For this review, use the dimensioned drawing (mm, ordinates from the lowest corner) and the shaded views. Give positions to 0.01 mm unless a question says otherwise; leave off trailing zeros. Loops run counter-clockwise (first coordinate to the right, second up) from the corner with the lowest first, then second, coordinate; pieces in that order, holes last. Notation, with made-up numbers: (-10, -8.5) -> (-1, -8.5) arc R33 ccw to (-1, 29.5) -> close; hole circle Ø3 at (87, 70.25). An arc over 180 degrees is marked (long way). Use a Markdown table: item, result. Add a question column.
1. For pin 1 Ø9 at (x, y) = (12.5, 12.5) entering from -Z; pin 2 Ø5 at (y, z) = (61, 3.5) entering from +X; pin 3 Ø5 at (x, z) = (83, 3) entering from -Y; pin 4 Ø6 at (y, z) = (18, 5.5) entering from -X, all flat-tipped, find the tip position at first contact; note any pin that passes through.
2. To check wall thickness, follow line 1 (Y direction, x = 12.5, z = 6.5); line 2 (X direction, y = 84, z = 7); line 3 (Y direction, x = 93, z = 3). State the ranges of each line that lie inside material, in increasing order.
3. Add section B-B (y = 87.5). State the section outline as (x, z) points, and give its area (3 significant figures).
4. Add section C-C (z = 6). State the section outline as (x, y) points (1 decimal), and give its area (3 significant figures).
5. Add section D-D (y = 12.5). State the section outline as (x, z) points.
6. Add section A-A (x = 12.5). State the section outline as (y, z) points, and give its area (3 significant figures).
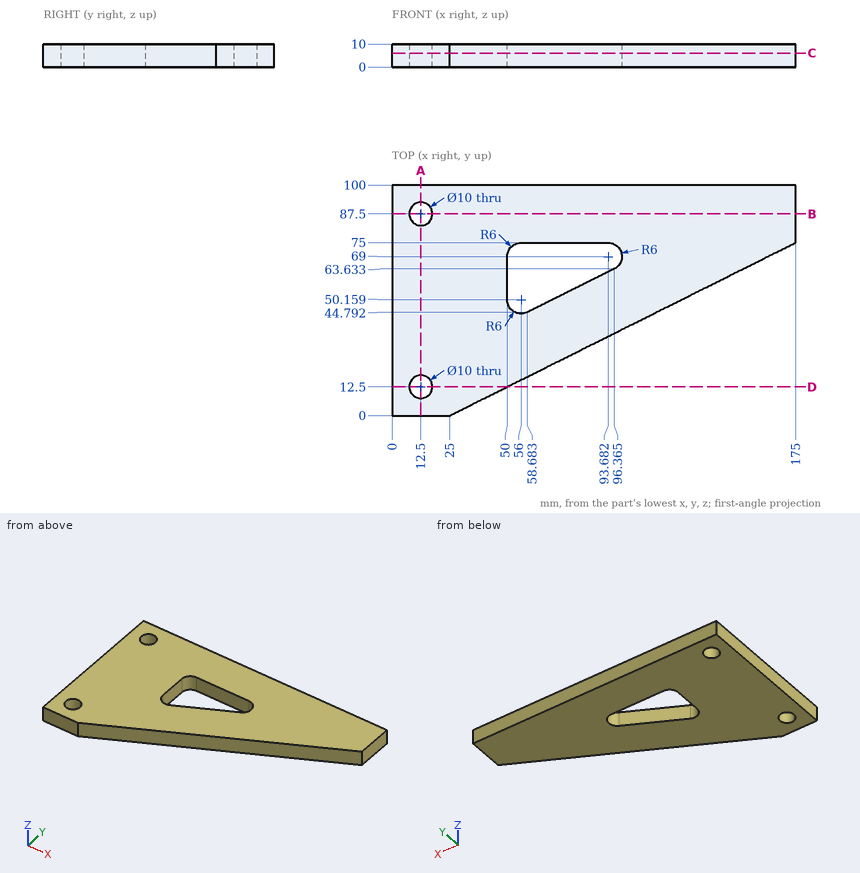
Taken from the geometry:
| question | item | result |
|---|---|---|
| 1 | pin 1 | passes through |
| 1 | pin 2 | stops at x = 152 |
| 1 | pin 3 | stops at y = 27.75 |
| 1 | pin 4 | stops at x = 0 |
| 2 | line 1 | y = 0 to 7.5, 17.5 to 82.5, 92.5 to 100 |
| 2 | line 2 | x = 0 to 8.93, 16.07 to 175 |
| 2 | line 3 | y = 34 to 61.95, 75 to 100 |
| 3 | outline | (0, 0) -> (7.5, 0) -> (7.5, 10) -> (0, 10) -> close; (17.5, 0) -> (175, 0) -> (175, 10) -> (17.5, 10) -> close |
| 3 | area | 1,650 mm^2 |
| 4 | outline | (0, 0) -> (25, 0) -> (175, 75) -> (175, 100) -> (0, 100) -> close; hole circle Ø10 at (12.5, 12.5); hole circle Ø10 at (12.5, 87.5); hole (50, 50.2) arc R6 ccw to (58.7, 44.8) -> (96.4, 63.6) arc R6 ccw to (93.7, 75) -> (56, 75) arc R6 ccw to (50, 69) -> close |
| 4 | area | 10,700 mm^2 |
| 5 | outline | (0, 0) -> (7.5, 0) -> (7.5, 10) -> (0, 10) -> close; (17.5, 0) -> (50, 0) -> (50, 10) -> (17.5, 10) -> close |
| 6 | outline | (0, 0) -> (7.5, 0) -> (7.5, 10) -> (0, 10) -> close; (17.5, 0) -> (82.5, 0) -> (82.5, 10) -> (17.5, 10) -> close; (92.5, 0) -> (100, 0) -> (100, 10) -> (92.5, 10) -> close |
| 6 | area | 800 mm^2 |
